Check sheet for the modelled part. Datum: model origin and axes. Units: mm. Face numbers are marked on the shaded views. A direction names the side the tool comes from. Round coordinates to 2 decimals unless told otherwise and drop trailing zeros. Write each loop counter-clockwise with the first axis right and the second up, starting at its lowest first coordinate (ties: lowest second). Pieces come first, ordered by that corner, then holes. Notation, with made-up numbers: M -4.5,77.25 L 26.5,77.25 A6 cw 26.5,83.25 Z; hole C 68,68 d9. An arc over 180 degrees is marked long. Put each result on its own line as item: value.
```python
from build123d import *

# Parameters (mm, degrees)
BOSS_EXTRUDE1_DEPTH = 2
BOSS_EXTRUDE2_DEPTH = 52
SKETCH4_R           = 1.6
CUT_EXTRUDE3_DEPTH  = 52
CUT_EXTRUDE4_DEPTH  = 52


with BuildPart() as part:
    # Sketch1 → Boss-Extrude1 (new body)
    with BuildSketch(Plane(origin=(0, 0, 0), x_dir=(1, 0, 0), z_dir=(0, 1, 0))):
        Polygon((0, 0), (-69.5, 0), (6.5, 103), (50, 0), (40, 0), align=None)
    extrude(amount=BOSS_EXTRUDE1_DEPTH)

    # Sketch2 → Boss-Extrude2 (add)
    with BuildSketch(Plane.XZ):
        Polygon((50, 0), (-69.5, 0), (6.5, -103), align=None)
        Polygon((5.786026753, -96.979592592), (45.476437216, -3), (-63.558138655, -3), align=None, mode=Mode.SUBTRACT)
    extrude(amount=BOSS_EXTRUDE2_DEPTH)

    # Sketch4 → Cut-Extrude3 (cut)
    with BuildSketch(Plane.XZ):
        with Locations((-39.790693273, -15)):
            Circle(SKETCH4_R)
        with Locations((27.382186082, -15)):
            Circle(SKETCH4_R)
        with Locations((2.930133764, -72.897962959)):
            Circle(SKETCH4_R)
    extrude(amount=-CUT_EXTRUDE3_DEPTH, mode=Mode.SUBTRACT)

    # Sketch6 → Cut-Extrude4 (cut)
    with BuildSketch(Plane.XZ.offset(52)):
        Polygon((5.786026753, -96.979592592), (13.566318251, -107.523935016), (48.733009709, -3), (45.476437216, -3), align=None)
    extrude(amount=-CUT_EXTRUDE4_DEPTH, mode=Mode.SUBTRACT)


solid = part.part
```
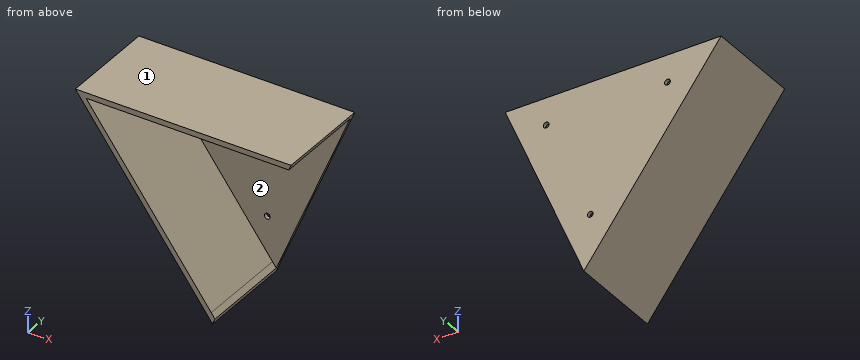
1. Scan lines: probe 1 along Y at (x, z) = (-4, -10); probe 2 along Z at (x, y) = (-51.5, -7.5); probe 3 along Z at (x, y) = (-38.5, -18.5). Record each from-to range of solid material in increasing order.
Computed values:
probe 1: y = 0 to 2
probe 2: z = -24.39 to -19.34, -3 to 0
probe 3: z = -42.01 to -36.96, -3 to 0
2. Cross-section at C-C (z = -50.5). Enter the section's corners in (x, y).
Computed values:
outline: M -32.24,-52 L -28.51,-52 L -28.51,0 L 28.67,0 L 28.67,2 L -32.24,2 Z
3. Cross-section at A-A (y = -17.5). Enter the section's corners in (x, z).
Computed values:
outline: M -69.5,0 L 6.5,-103 L 7.86,-99.79 L -63.56,-3 L 48.73,-3 L 50,0 Z
4. Cross-section at D-D (z = -92.5). Enter the section's corners in (x, y).
Computed values:
outline: M -1.25,-52 L 2.48,-52 L 2.48,0 L 10.93,0 L 10.93,2 L -1.25,2 Z
5. Depth check by flat-ended pin: pin 1 Ø4 at (x, z) = (-21.5, -59) entering from -Y; pin 2 Ø1.5 at (y, z) = (-15, -76.5) entering from -X; pin 3 Ø2 at (x, z) = (1, -11) entering from -Y; pin 4 Ø6 at (y, z) = (-39, -48.5) entering from +X. Enter the tip coordinate at first touch or a pass-through.
Computed values:
pin 1: stops at y = -52
pin 2: stops at x = -13.61
pin 3: stops at y = 0
pin 4: stops at x = -27.77
6. Cross-section at B-B (z = -15). Enter the section's corners in (x, y), then the cut area to 3 significant figures.
Computed values:
outline: M -58.43,-52 L -54.7,-52 L -54.7,0 L -41.39,0 L -41.39,2 L -58.43,2 Z; M -38.19,0 L 25.78,0 L 25.78,2 L -38.19,2 Z; M 28.98,0 L 43.67,0 L 43.67,2 L 28.98,2 Z
area: 385 mm2
7. Access from +Z, -Z, +X, -X, +Y, -Y to the whole of each face (thin tool, end or side, straight path). Record for the marked faces 1 and 2.
Computed values:
face 1: +Z, +X, -X, +Y, -Y
face 2: +X, -Y
